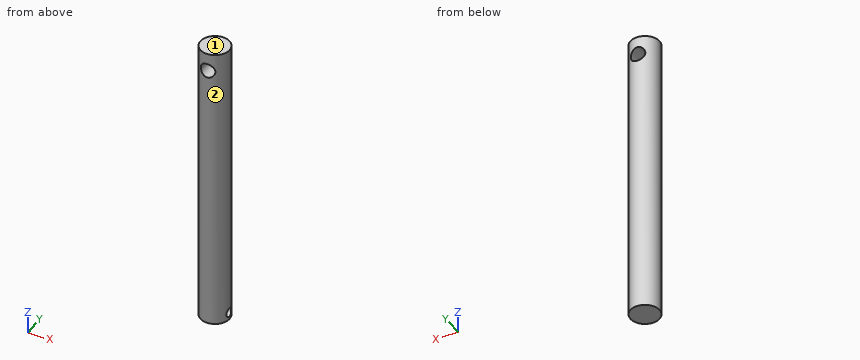
```python
from build123d import *

# Parameters (mm, degrees)
SKETCH_1_R               = 8
EXTRUDE_1_DEPTH          = 160
SKETCH_2_R               = 4
CUT_EXTRUDE_1_DEPTH      = 120
CUT_EXTRUDE_1_DEPTH_BACK = 120
SKETCH_3_R               = 2.5
CUT_EXTRUDE_2_DEPTH      = 10


with BuildPart() as part:
    # Sketch 1 → Extrude 1 (new body)
    with BuildSketch(Plane.XY):
        Circle(SKETCH_1_R)
    extrude(amount=EXTRUDE_1_DEPTH)

    # Sketch 2 → Cut-Extrude 1 (cut, two sides)
    with BuildSketch(Plane(origin=(0, 0, 0), x_dir=(1, 0, 0), z_dir=(0, 1, 0))) as cut_extrude_1_sk:
        with Locations((0, -150)):
            Circle(SKETCH_2_R)
    extrude(amount=CUT_EXTRUDE_1_DEPTH, mode=Mode.SUBTRACT)
    extrude(cut_extrude_1_sk.sketch, amount=-CUT_EXTRUDE_1_DEPTH_BACK, mode=Mode.SUBTRACT)

    # Sketch 3 → Cut-Extrude 2 (cut)
    with BuildSketch(Plane(origin=(0, 0, 0), x_dir=(0, 0, -1), z_dir=(1, 0, 0))):
        with Locations((-4, 0)):
            Circle(SKETCH_3_R)
    extrude(amount=CUT_EXTRUDE_2_DEPTH, mode=Mode.SUBTRACT)


solid = part.part
```
Input: part model. Units: mm. Frame: model coordinates. Face numbers are marked on the shaded views. Coordinates: 2 decimals unless noted, no trailing zeros. Write each loop counter-clockwise with the first axis right and the second up, starting at its lowest first coordinate (ties: lowest second). Pieces come first, ordered by that corner, then holes. Notation, with made-up numbers: (87, -28) -> (134, -28) arc R27 ccw to (134, -6) -> close; hole circle Ø4 at (2, 65.25). An arc over 180 degrees is marked (long way). Answer as a JSON object with one key per item and string values.
1. Material intervals for line 1 (Z direction, x = 0, y = -3.5); line 2 (X direction, y = 6.25, z = 150); line 3 (Z direction, x = -2.25, y = -6.5), sorted ascending. Write a range as from..to.
Result set:
{"line 1": "z = 0..146, 154..160", "line 2": "x = -4.99..-4, 4..4.99", "line 3": "z = 0..146.69, 153.31..160"}
2. Section A-A on y = -5. Return the cut outline in (x, z) (3 decimals), then the cut area to 3 significant figures.
Result set:
{"outline": "(-6.245, 0) -> (6.245, 0) -> (6.245, 160) -> (-6.245, 160) -> close; hole circle Ø8 at (0, 150)", "area": "1,950 mm2"}
3. Section D-D on z = 4. Return the cut outline in (x, y).
Result set:
{"outline": "(0, -2.5) -> (0, 2.5) -> (7.6, 2.5) arc R8 ccw (long way) to (7.6, -2.5) -> close"}
4. Mould query, pull axis Y, two halves, no side actions, for the marked faces 1 and 2. Classes: released by +Y, released by -Y, zero draft, split by the parting line, or undercut.
Result set:
{"face 1": "zero draft", "face 2": "split by the parting line"}
5. Section C-C on z = 150. Return the cut outline in (x, y), then the cut area to 3 significant figures.
Result set:
{"outline": "(-4, -6.93) -> (-4, 6.93) arc R8 ccw to start; (4, -6.93) arc R8 ccw to (4, 6.93) -> close", "area": "78.6 mm2"}
6. Section B-B on z = 41.5. Return the cut outline in (x, y), then the cut area to 3 significant figures.
Result set:
{"outline": "circle Ø16 at (0, 0)", "area": "201 mm2"}
